```python
from build123d import *

# Parameters (mm, degrees)
F1_DEPTH = 5
F2_R     = 2.5
F2_R_2   = 1.5
F3_DEPTH = 2
F4_R     = 15
F5_DEPTH = 25
F6_DEPTH = 25


with BuildPart() as f1:
    # F0 (on Top) → F1 (new body)
    with BuildSketch(Plane.XY):
        with BuildLine():
            Line((-8.5, 0), (-8.5, 39.0864426624))
            ThreePointArc((-8.5, 39.0864426624), (-40, 0), (-8.5, -39.0864426624))
            Line((-8.5, -39.0864426624), (-8.5, 0))
        make_face()
        with BuildLine():
            ThreePointArc((0, -40), (4.2744761962, -39.7709548948), (8.5, -39.0864426624))
            Line((8.5, -39.0864426624), (8.5, 0))
            Line((8.5, 0), (0, 0))
            Line((0, 0), (-8.5, 0))
            Line((-8.5, 0), (-8.5, -39.0864426624))
            ThreePointArc((-8.5, -39.0864426624), (-4.2744761962, -39.7709548948), (0, -40))
        make_face()
        with BuildLine():
            ThreePointArc((2.5, -35), (1.767766953, -36.767766953), (0, -37.5))
            ThreePointArc((0, -37.5), (-1.767766953, -33.232233047), (2.5, -35))
        make_face(mode=Mode.SUBTRACT)
        with BuildLine():
            Line((8.5, 0), (8.5, 39.0864426624))
            ThreePointArc((8.5, 39.0864426624), (4.2744761962, 39.7709548948), (0, 40))
            ThreePointArc((0, 40), (-4.2744761962, 39.7709548948), (-8.5, 39.0864426624))
            Line((-8.5, 39.0864426624), (-8.5, 0))
            Line((-8.5, 0), (0, 0))
            Line((0, 0), (8.5, 0))
        make_face()
        with BuildLine():
            ThreePointArc((2.5, 35), (-1.767766953, 33.232233047), (0, 37.5))
            ThreePointArc((0, 37.5), (1.767766953, 36.767766953), (2.5, 35))
        make_face(mode=Mode.SUBTRACT)
        with BuildLine():
            ThreePointArc((8.5, -39.0864426624), (31.1448230048, -25.099800796), (40, 0))
            ThreePointArc((40, 0), (31.1448230048, 25.099800796), (8.5, 39.0864426624))
            Line((8.5, 39.0864426624), (8.5, 0))
            Line((8.5, 0), (8.5, -39.0864426624))
        make_face()
        with BuildLine():
            ThreePointArc((2.5, 35), (1.767766953, 36.767766953), (0, 37.5))
            ThreePointArc((0, 37.5), (-1.767766953, 33.232233047), (2.5, 35))
        make_face()
        with BuildLine():
            ThreePointArc((1.5, 35), (-1.0606601718, 33.9393398282), (0, 36.5))
            ThreePointArc((0, 36.5), (1.0606601718, 36.0606601718), (1.5, 35))
        make_face(mode=Mode.SUBTRACT)
        with BuildLine():
            ThreePointArc((2.5, -35), (-1.767766953, -33.232233047), (0, -37.5))
            ThreePointArc((0, -37.5), (1.767766953, -36.767766953), (2.5, -35))
        make_face()
        with BuildLine():
            ThreePointArc((1.5, -35), (1.0606601718, -36.0606601718), (0, -36.5))
            ThreePointArc((0, -36.5), (-1.0606601718, -33.9393398282), (1.5, -35))
        make_face(mode=Mode.SUBTRACT)
    extrude(amount=F1_DEPTH)

    # F2 (on face) → F3 (cut)
    with BuildSketch(Plane.XY.offset(5)):
        with Locations((0, 35)):
            Circle(F2_R)
        with Locations((0, 35)):
            Circle(F2_R_2, mode=Mode.SUBTRACT)
        with Locations((0, -35)):
            Circle(F2_R)
        with Locations((0, -35)):
            Circle(F2_R_2, mode=Mode.SUBTRACT)
    extrude(amount=-F3_DEPTH, mode=Mode.SUBTRACT)

    # F4 (on face) → F5 (cut)
    with BuildSketch(Plane.XY.offset(5)):
        Circle(F4_R)
    extrude(amount=-F5_DEPTH, mode=Mode.SUBTRACT)

    # F6 (cut): faces of the model
    f6_faces = [f1.faces().sort_by_distance(p)[0] for p in [
        (-2.4292893219, 35, 3),
        (-2.4292893219, -35, 3),
    ]]
    extrude(f6_faces, amount=-F6_DEPTH, mode=Mode.SUBTRACT)


solid = f1.part
```
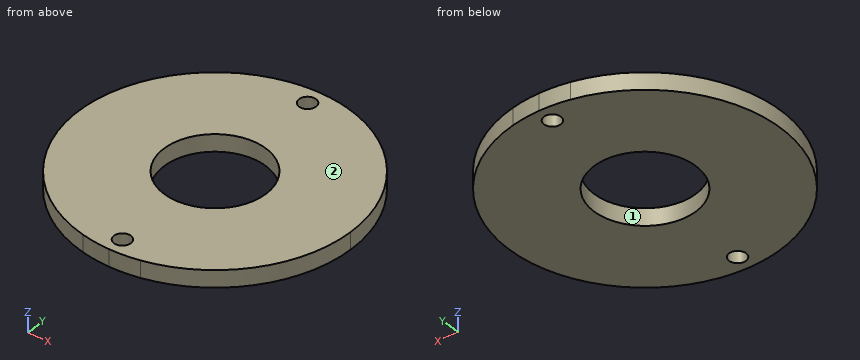
Check sheet for the modelled part. Datum: model origin and axes. Units: mm. Face numbers are marked on the shaded views. Round coordinates to 2 decimals unless told otherwise and drop trailing zeros. Loops run counter-clockwise (first coordinate to the right, second up) from the corner with the lowest first, then second, coordinate; pieces in that order, holes last. Notation, with made-up numbers: (2.25, 10) -> (33.25, 10) arc R34 ccw to (33.25, 48) -> close; hole circle Ø7 at (83.25, 86.5). An arc over 180 degrees is marked (long way). Answer in a Markdown table with one row per item.
Q1. Release check for a two-part mould opening along X. For the marked faces 1 and 2 record: released by +X, released by -X, zero draft, split by the parting line, or undercut.
Data:
| item | result |
|---|---|
| face 1 | undercut |
| face 2 | zero draft |
Q2. Go/stop test with flat-tipped pins: P1, Ø2, axis at x = 27.5, z = 3, coming from the +Y side; P2, Ø2, axis at x = -4.5, z = 4, coming from the +Y side; P3, Ø1.5, axis at x = 31, z = 3.5, coming from the -Y side. Record where each tip stops, or that it passes through.
Data:
| item | result |
|---|---|
| P1 | stops at y = 29.96 |
| P2 | stops at y = 39.85 |
| P3 | stops at y = -26.17 |
Q3. Sectioned sample at B-B on y = 8. Enter the section's corners in (x, z).
Data:
| item | result |
|---|---|
| outline | (-39.19, 0) -> (-12.69, 0) -> (-12.69, 5) -> (-39.19, 5) -> close; (12.69, 0) -> (39.19, 0) -> (39.19, 5) -> (12.69, 5) -> close |
Q4. Sectioned sample at C-C on x = 1. Enter the section's corners in (y, z).
Data:
| item | result |
|---|---|
| outline | (-39.99, 0) -> (-37.29, 0) -> (-37.29, 5) -> (-39.99, 5) -> close; (-32.71, 0) -> (-14.97, 0) -> (-14.97, 5) -> (-32.71, 5) -> close; (14.97, 0) -> (32.71, 0) -> (32.71, 5) -> (14.97, 5) -> close; (37.29, 0) -> (39.99, 0) -> (39.99, 5) -> (37.29, 5) -> close |
Q5. Sectioned sample at A-A on z = 1.4. Enter the section's corners in (x, y).
Data:
| item | result |
|---|---|
| outline | circle Ø80 at (0, 0); hole circle Ø30 at (0, 0); hole circle Ø5 at (0, -35); hole circle Ø5 at (0, 35) |
Q6. Thickness scan on L1, parallel to X at y = -13.5, z = 0.6; L2, parallel to X at y = 3.5, z = 4.25; L3, parallel to Y at x = 10, z = 0.8. Record the ranges inside material, lowest first.
Data:
| item | result |
|---|---|
| L1 | x = -37.65 to -6.54, 6.54 to 37.65 |
| L2 | x = -39.85 to -14.59, 14.59 to 39.85 |
| L3 | y = -38.73 to -11.18, 11.18 to 38.73 |
Q7. Sectioned sample at D-D on x = 32. Enter the section's corners in (y, z), then the cut area to 3 significant figures.
Data:
| item | result |
|---|---|
| outline | (-24, 0) -> (24, 0) -> (24, 5) -> (-24, 5) -> close |
| area | 240 mm^2 |
